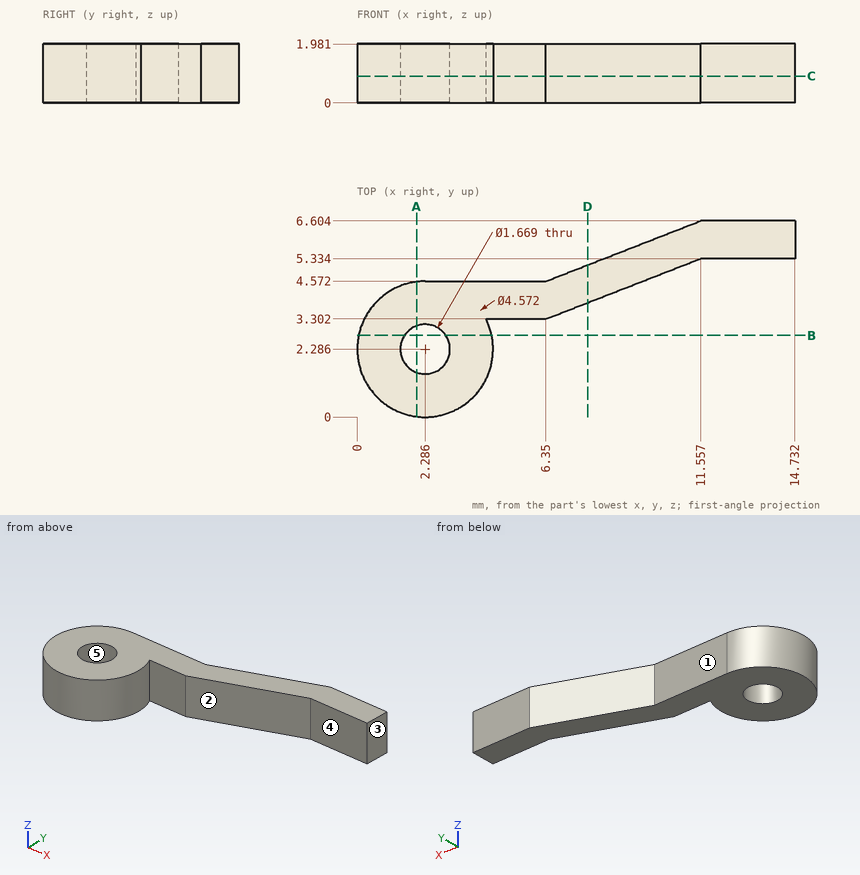
Design review of the part shown in the three views and the two pictorial views. Dimensions are in mm from the part's minimum x, y and z. A direction names the side the tool comes from. Round coordinates to 2 decimals unless told otherwise and drop trailing zeros. Loops run counter-clockwise (first coordinate to the right, second up) from the corner with the lowest first, then second, coordinate; pieces in that order, holes last.
(1) Wall thickness on line 1 along Y through (x, z) = (12.5, 0.3); line 2 along Y through (x, z) = (2.75, 1.7); line 3 along Y through (x, z) = (1.75, 0.15) (1 decimal): over which ranges is each line inside the solid? List them lowest first.
Returned:
line 1: y = 5.33 to 6.6
line 2: y = 0.05 to 1.59, 2.98 to 4.57
line 3: y = 0.1 to 1.6, 2.9 to 4.5
(2) Tool access review of the marked faces 1 and 2: name each direction out of +Z, -Z, +X, -X, +Y, -Y from which nothing blocks a thin tool from reaching the whole face with its end or side.
Returned:
face 1: +Z, -Z, -X, +Y
face 2: +Z, -Z, +X, -Y
(3) Clearance check with flat-ended pins moving along their axes: P1, Ø0.6, axis at x = 13, z = 0.5, coming from the -Y side; P2, Ø1.5, axis at x = 2.29, y = 2.29, coming from the +Z side. State where each tip first meets the part, or that it passes through.
Returned:
P1: stops at y = 5.33
P2: passes through
(4) Mouldability with a two-part tool opening along Y and no side actions: class the marked faces 3, 4 and 5 as released by +Y, released by -Y, zero draft, split by the parting line, or undercut.
Returned:
face 3: zero draft
face 4: released by -Y
face 5: undercut
(5) We need section C-C (z = 0.9). Give the boundary of the cut face in (x, y).
Returned:
outline: (2.29, 4.57) arc R2.29 ccw (long way) to (4.33, 3.3) - (6.35, 3.3) - (11.56, 5.33) - (14.73, 5.33) - (14.73, 6.6) - (11.56, 6.6) - (6.35, 4.57) - close; hole circle Ø1.67 at (2.29, 2.29)
(6) We need section A-A (x = 2). Give the boundary of the cut face in (y, z).
Returned:
outline: (0.02, 0) - (1.5, 0) - (1.5, 1.98) - (0.02, 1.98) - close; (3.07, 0) - (4.55, 0) - (4.55, 1.98) - (3.07, 1.98) - close
(7) We need section B-B (y = 2.75). Give the boundary of the cut face in (x, z).
Returned:
outline: (0.05, 0) - (1.59, 0) - (1.59, 1.98) - (0.05, 1.98) - close; (2.98, 0) - (4.52, 0) - (4.52, 1.98) - (2.98, 1.98) - close
(8) We need section D-D (x = 7.75). Give the boundary of the cut face in (y, z).
Returned:
outline: (3.85, 0) - (5.12, 0) - (5.12, 1.98) - (3.85, 1.98) - close
